```python
from build123d import *

# Parameters (mm, degrees)
BOSS_EXTRUDE1_DEPTH     = 29
CUT_EXTRUDE1_START      = -1.5
CUT_EXTRUDE1_DEPTH      = 55
BOSS_EXTRUDE2_DEPTH     = 0.5
CUT_EXTRUDE2_DEPTH      = 42.303752856
CUT_EXTRUDE2_DEPTH_BACK = 42.303752856
SKETCH5_W               = 8.5
SKETCH5_H               = 17
SKETCH6_W               = 6
SKETCH6_H               = 2
CUT_EXTRUDE3_DEPTH      = 10
SKETCH7_R               = 1.5
CUT_EXTRUDE4_DEPTH      = 10
CUT_EXTRUDE5_START      = -10
SKETCH8_R               = 1.5
CUT_EXTRUDE5_DEPTH      = 10
SKETCH9_R               = 1.6
CUT_EXTRUDE6_DEPTH      = 42.303752856


with BuildPart() as part:
    # Sketch2 → Boss-Extrude1 (new, symmetric)
    with BuildSketch(Plane(origin=(0, 0, 0), x_dir=(1, 0, 0), z_dir=(0, 1, 0))):
        with BuildLine():
            Line((24, 0), (-24, 0))
            Line((-24, 0), (-24, -8))
            ThreePointArc((-24, -8), (-21.363961031, -14.363961031), (-15, -17))
            Line((-15, -17), (15, -17))
            ThreePointArc((15, -17), (21.363961031, -14.363961031), (24, -8))
            Line((24, -8), (24, 0))
        make_face()
    extrude(amount=BOSS_EXTRUDE1_DEPTH, both=True)

    # Sketch3 → Cut-Extrude1 (cut)
    with BuildSketch(Plane.XZ.offset(29).offset(CUT_EXTRUDE1_START)):
        with BuildLine():
            Line((-14.319593213, 17.6), (14.319593213, 17.6))
            ThreePointArc((14.319593213, 17.6), (20.457567716, 15.057567716), (23, 8.919593213))
            Line((23, 8.919593213), (23, 1))
            Line((23, 1), (-23, 1))
            Line((-23, 1), (-23, 8.919593213))
            ThreePointArc((-23, 8.919593213), (-20.457567716, 15.057567716), (-14.319593213, 17.6))
        make_face()
    extrude(amount=-CUT_EXTRUDE1_DEPTH, mode=Mode.SUBTRACT)

    # Sketch4 → Boss-Extrude2 (add, symmetric)
    with BuildSketch(Plane(origin=(7.75, 0, 0), x_dir=(0, 0, -1), z_dir=(1, 0, 0))):
        Polygon((-16, 27.5), (-1, 27.5), (-1, -27.5), (-16, -27.5), (-8, -17), (-8, 17), align=None)
    boss_extrude2 = extrude(amount=BOSS_EXTRUDE2_DEPTH, both=True)

    # Mirror1: Boss-Extrude2 across plane
    add(boss_extrude2.mirror(Plane(origin=(0, 0, 0), x_dir=(0, 0, 1), z_dir=(1, 0, 0))))

    # Sketch5 → Cut-Extrude2 (cut, two sides: drawn at the far end of the back side and taken through both)
    with BuildSketch(Plane(origin=(0, 0, 0), x_dir=(0, 0, -1), z_dir=(1, 0, 0)).offset(-CUT_EXTRUDE2_DEPTH_BACK)):
        with Locations((-12.75, 0)):
            Rectangle(SKETCH5_W, SKETCH5_H)
    extrude(amount=CUT_EXTRUDE2_DEPTH + CUT_EXTRUDE2_DEPTH_BACK, mode=Mode.SUBTRACT)

    # Sketch6 → Cut-Extrude3 (cut)
    with BuildSketch(Plane(origin=(24, 0, 0), x_dir=(0, 0, -1), z_dir=(1, 0, 0))):
        with Locations((-14, 26.5)):
            Rectangle(SKETCH6_W, SKETCH6_H)
        with Locations((-14, -26.5)):
            Rectangle(SKETCH6_W, SKETCH6_H)
    cut_extrude3 = extrude(amount=-CUT_EXTRUDE3_DEPTH, mode=Mode.SUBTRACT)

    # Mirror2: Cut-Extrude3 across plane
    add(cut_extrude3.mirror(Plane(origin=(0, 0, 0), x_dir=(0, 0, 1), z_dir=(1, 0, 0))), mode=Mode.SUBTRACT)

    # Sketch7 → Cut-Extrude4 (cut)
    with BuildSketch(Plane(origin=(0, 29, 0), x_dir=(1, 0, 0), z_dir=(0, 1, 0))):
        with Locations(Location((-15, -10, 0), (0, 0, 270))):
            Circle(SKETCH7_R)
        with Locations(Location((0, -10, 0), (0, 0, 270))):
            Circle(SKETCH7_R)
        with Locations(Location((15, -10, 0), (0, 0, 270))):
            Circle(SKETCH7_R)
    extrude(amount=-CUT_EXTRUDE4_DEPTH, mode=Mode.SUBTRACT)

    # Sketch8 → Cut-Extrude5 (cut)
    with BuildSketch(Plane.XZ.offset(29).offset(CUT_EXTRUDE5_START)):
        with Locations(Location((-15, 10, 0), (0, 0, 90))):
            Circle(SKETCH8_R)
        with Locations(Location((15, 10, 0), (0, 0, 90))):
            Circle(SKETCH8_R)
        with Locations(Location((-1.5, 10, 0), (0, 0, 270))):
            Circle(SKETCH8_R)
    extrude(amount=CUT_EXTRUDE5_DEPTH, mode=Mode.SUBTRACT)

    # Sketch9 → Cut-Extrude6 (cut, through all)
    with BuildSketch(Plane(origin=(0, 0, 0), x_dir=(-1, 0, 0), z_dir=(0, 0, -1))):
        with Locations((-15, 0)):
            Circle(SKETCH9_R)
        with Locations((15, 0)):
            Circle(SKETCH9_R)
    extrude(amount=-CUT_EXTRUDE6_DEPTH, mode=Mode.SUBTRACT)


solid = part.part
```
Check sheet for the modelled part. Datum: model origin and axes. Units: mm. A direction names the side the tool comes from. Coordinates: 2 decimals unless noted, no trailing zeros. Write each loop counter-clockwise with the first axis right and the second up, starting at its lowest first coordinate (ties: lowest second). Pieces come first, ordered by that corner, then holes. Notation, with made-up numbers: (-35.75, 17.25) - (4.25, 17.25) arc R14 ccw to (4.25, 27.25) - close; hole circle Ø10 at (68.25, -8). An arc over 180 degrees is marked (long way). One line per question, with ' | ' between items.
Item 1: Mould release check, pull along X, two halves, no side actions. Record for faces 4 (the face through (16.6, 0.07, 0.49)), 5 (the face through (-22.4, 25.5, 12.6)), 6 (the face through (23.114, -12.483, 11.893)): pulls with the +X half, pulls with the -X half, needs draft (parallel to the pull), parting line crosses it, or undercut.
Determined:
face 4: undercut | face 5: needs draft | face 6: pulls with the +X half
Item 2: Sectioned sample at A-A on y = 0. Record the boundary of the cut face in (x, z), plus the area to 3 significant figures.
Determined:
outline: (-24, 0) - (-16.6, 0) - (-16.6, 1) - (-23, 1) - (-23, 8.5) - (-23.99, 8.5) arc R9 ccw to (-24, 8) - close; (-13.4, 0) - (13.4, 0) - (13.4, 1) - (8.25, 1) - (8.25, 8) - (7.25, 8) - (7.25, 1) - (-7.25, 1) - (-7.25, 8) - (-8.25, 8) - (-8.25, 1) - (-13.4, 1) - close; (16.6, 0) - (24, 0) - (24, 8) arc R9 ccw to (23.99, 8.5) - (23, 8.5) - (23, 1) - (16.6, 1) - close | area: 70.6 mm2
Item 3: Sectioned sample at B-B on z = 2. Record the boundary of the cut face in (x, y), plus the area to 3 significant figures.
Determined:
outline: (-24, -29) - (24, -29) - (24, 29) - (-24, 29) - close; hole (-23, -27.5) - (-8.25, -27.5) - (-8.25, 27.5) - (-23, 27.5) - close; hole (-7.25, -27.5) - (7.25, -27.5) - (7.25, 27.5) - (-7.25, 27.5) - close; hole (8.25, -27.5) - (23, -27.5) - (23, 27.5) - (8.25, 27.5) - close | area: 364 mm2
Item 4: Sectioned sample at D-D on y = 24.5. Record the boundary of the cut face in (x, z), plus the area to 3 significant figures.
Determined:
outline: (-24, 0) - (24, 0) - (24, 8) arc R9 ccw to (20, 15.48) arc R8.68 cw to (23, 8.92) - (23, 1) - (8.25, 1) - (8.25, 13.71) - (7.25, 13.71) - (7.25, 1) - (-7.25, 1) - (-7.25, 13.71) - (-8.25, 13.71) - (-8.25, 1) - (-23, 1) - (-23, 8.92) arc R8.68 cw to (-20, 15.48) arc R9 ccw to (-24, 8) - close | area: 96.7 mm2
Item 5: Thickness scan on line 1 (X direction, y = 0, z = 6.5); line 2 (Y direction, x = 12.5, z = 15.25); line 3 (X direction, y = 28.2, z = 10). Record the ranges inside material, lowest first. Write a range as [from, to].
Determined:
line 1: x = [-24, -23], [-8.25, -7.25], [7.25, 8.25], [23, 24] | line 2: y = [-29, -27.5], [27.5, 29] | line 3: x = [-23.77, -16.5], [-13.5, -1.5], [1.5, 13.5], [16.5, 23.77]
Item 6: Access from +Z, -Z, +X, -X, +Y, -Y to the whole of each face (thin tool, end or side, straight path). Record for faces 1 (the face through (-23, 8.5, 11)), 2 (the face through (-22.236, 17.867, 12.481)), 3 (the face through (-8.25, 0, 5)).
Determined:
face 1: +Z, +X, -X | face 2: none | face 3: +Z
Item 7: Gauge pin test, flat ends, axial feed: P1, Ø4, axis at x = 0, z = 10, coming from the +Y side; P2, Ø10, axis at y = 12.5, z = 14.5, coming from the -X side; P3, Ø0.8, axis at x = 23.5, y = 0, coming from the +Z side; P4, Ø0.8, axis at x = 7.5, y = -7.5, coming from the +Z side. Record the tip position at first contact, or that the pin passes through.
Determined:
P1: stops at y = 29 | P2: stops at x = -23.87 | P3: stops at z = 8.5 | P4: stops at z = 8
Item 8: Sectioned sample at C-C on x = -4. Record the boundary of the cut face in (y, z).
Determined:
outline: (-29, 0) - (29, 0) - (29, 17) - (27.5, 17) - (27.5, 1) - (-27.5, 1) - (-27.5, 17) - (-29, 17) - close
